Input: part model. Units: mm. Frame: model coordinates. Round coordinates to 2 decimals unless told otherwise and drop trailing zeros. Loops run counter-clockwise (first coordinate to the right, second up) from the corner with the lowest first, then second, coordinate; pieces in that order, holes last.
1) Section C-C, the plane y = 0.5. State how many separate pieces and enclosed holes the cut face has, and give its area (3 significant figures).
2) Ray query, line 1 along Z through (x, y) = (-41, 0.6); line 2 along X through (y, z) = (1.55, 247.5); line 3 along X through (y, z) = (1.05, 193.5). Return the intervals inside material, ascending.
3) First-contact query: pin 1 (0.5 mm diameter, centred on x = -77, y = 0.5, fed in from -Z); pin 2 (4 mm diameter, centred on x = -41.78, z = 255.06, fed in from -Y). Flat tips, straight axial feed; report the tip coordinate or a pass-through.
4) Section B-B, the plane z = 62. Return loops of the section in (x, y), and give its area (3 significant figures).
5) Section A-A, the plane x = -80. Return loops of the section in (y, z), and give its area (3 significant figures).
from build123d import *

# Parameters (mm, degrees)
SKETCH1_R        = 1.5
SKETCH1_R_2      = 1.600010398
SKETCH1_R_3      = 1.6
SKETCH1_R_4      = 1.35
EXTRUSION1_DEPTH = 1.6
FILLET1_R        = 1
FILLET2_R        = 4
FILLET3_R        = 3
FILLET4_R        = 3
FILLET5_R        = 2
FILLET6_R        = 2
FILLET7_R        = 3
FILLET8_R        = 3
FILLET9_R        = 2
FILLET10_R       = 2
FILLET11_R       = 3


with BuildPart() as part:
    # Sketch1 → Extrusion1 (new body)
    with BuildSketch(Plane(origin=(0, 0, 0), x_dir=(-1, 0, 0), z_dir=(0, 1, 0))):
        Polygon((59.775158519, 259.059874387), (56.775158519, 264.05987395), (36.775158519, 264.05987395), (36.775158519, 252.05987395), (18.755330752, 234.731117294), (21.527931817, 231.847944851), (10.275158581, 204.559863083), (7.271137723, 204.559863083), (7.157131709, 183.059873956), (7.157131709, 76.612413837), (10.15713177, 76.612413837), (21.409905007, 49.324332069), (18.637303942, 46.441159626), (36.657131709, 29.11240297), (36.657131709, 17.11240297), (56.657131709, 17.11240297), (59.657131709, 22.112402533), (78.657131709, 22.112402533), (97.657131709, 22.112402533), (100.657131709, 17.11240297), (120.657131709, 17.11240297), (120.657131709, 29.11240297), (138.676959475, 46.441159626), (135.90435841, 49.324332069), (147.157131647, 76.612413837), (150.157131709, 76.612413837), (150.157131709, 183.059873956), (150.275158519, 204.559863083), (147.275158457, 204.559863083), (136.022385221, 231.847944851), (138.794986286, 234.731117294), (120.775158519, 252.05987395), (120.775158519, 264.05987395), (100.775158519, 264.05987395), (97.775158519, 259.059874387), (78.657131709, 259.059874387), align=None)
        with Locations((55.657131647, 26.112401639)):
            Circle(SKETCH1_R, mode=Mode.SUBTRACT)
        with Locations((39.157131647, 33.112413837)):
            Circle(SKETCH1_R, mode=Mode.SUBTRACT)
        with Locations((53.657131709, 208.059873956)):
            Circle(SKETCH1_R_2, mode=Mode.SUBTRACT)
        with Locations((53.657131709, 158.059873956)):
            Circle(SKETCH1_R_2, mode=Mode.SUBTRACT)
        with Locations((17.157131647, 89.862401639)):
            Circle(SKETCH1_R_3, mode=Mode.SUBTRACT)
        with Locations((103.657131709, 158.059873956)):
            Circle(SKETCH1_R_2, mode=Mode.SUBTRACT)
        with Locations((41.775158457, 255.059863083)):
            Circle(SKETCH1_R, mode=Mode.SUBTRACT)
        with Locations((39.275158457, 248.059863083)):
            Circle(SKETCH1_R, mode=Mode.SUBTRACT)
        with Locations((10.775158457, 194.05987528)):
            Circle(SKETCH1_R_4, mode=Mode.SUBTRACT)
        with Locations((88.65713177, 26.862413837)):
            Circle(SKETCH1_R, mode=Mode.SUBTRACT)
        with Locations((115.65713177, 26.112413837)):
            Circle(SKETCH1_R, mode=Mode.SUBTRACT)
        with Locations((118.15713177, 33.112413837)):
            Circle(SKETCH1_R, mode=Mode.SUBTRACT)
        with Locations((140.15713177, 89.862401639)):
            Circle(SKETCH1_R_3, mode=Mode.SUBTRACT)
        with Locations((115.775158581, 255.059863083)):
            Circle(SKETCH1_R, mode=Mode.SUBTRACT)
        with Locations((88.775158581, 254.309863083)):
            Circle(SKETCH1_R, mode=Mode.SUBTRACT)
        with Locations((140.275158581, 191.30987528)):
            Circle(SKETCH1_R_3, mode=Mode.SUBTRACT)
        with Locations((146.775158581, 194.05987528)):
            Circle(SKETCH1_R_4, mode=Mode.SUBTRACT)
        with Locations((101.775158581, 255.05987528)):
            Circle(SKETCH1_R, mode=Mode.SUBTRACT)
        with Locations((118.275158581, 248.059863083)):
            Circle(SKETCH1_R, mode=Mode.SUBTRACT)
        with Locations((146.65713177, 87.112401639)):
            Circle(SKETCH1_R_4, mode=Mode.SUBTRACT)
        with Locations((101.65713177, 26.112401639)):
            Circle(SKETCH1_R, mode=Mode.SUBTRACT)
        with Locations((17.275158457, 191.30987528)):
            Circle(SKETCH1_R_3, mode=Mode.SUBTRACT)
        with Locations((55.775158457, 255.05987528)):
            Circle(SKETCH1_R, mode=Mode.SUBTRACT)
        with Locations((68.775158457, 254.309863083)):
            Circle(SKETCH1_R, mode=Mode.SUBTRACT)
        with Locations((10.657131647, 87.112401639)):
            Circle(SKETCH1_R_4, mode=Mode.SUBTRACT)
        with Locations((68.657131647, 26.862413837)):
            Circle(SKETCH1_R, mode=Mode.SUBTRACT)
        with Locations((41.657131647, 26.112413837)):
            Circle(SKETCH1_R, mode=Mode.SUBTRACT)
        with Locations((32.657131647, 39.362413837)):
            Circle(SKETCH1_R, mode=Mode.SUBTRACT)
        with Locations((124.775158581, 241.809863083)):
            Circle(SKETCH1_R, mode=Mode.SUBTRACT)
        with Locations((32.775158457, 241.809863083)):
            Circle(SKETCH1_R, mode=Mode.SUBTRACT)
        with Locations((103.657131709, 208.059873956)):
            Circle(SKETCH1_R_2, mode=Mode.SUBTRACT)
        with Locations((124.65713177, 39.362413837)):
            Circle(SKETCH1_R, mode=Mode.SUBTRACT)
    extrude(amount=EXTRUSION1_DEPTH)

    # Fillet1
    fillet1_edges = [part.edges().sort_by_distance(p)[0] for p in [
        (-97.775158519, 0.8, 259.059874387),
        (-97.657131709, 0.8, 22.112402533),
        (-59.657131709, 0.8, 22.112402533),
        (-59.775158519, 0.8, 259.059874387),
    ]]
    fillet(fillet1_edges, radius=FILLET1_R)

    # Fillet2
    fillet2_edges = [part.edges().sort_by_distance(p)[0] for p in [
        (-120.775158519, 0.8, 264.05987395),
        (-120.657131709, 0.8, 17.11240297),
        (-36.657131709, 0.8, 17.11240297),
        (-36.775158519, 0.8, 264.05987395),
    ]]
    fillet(fillet2_edges, radius=FILLET2_R)

    # Fillet3
    fillet3_edges = [part.edges().sort_by_distance(p)[0] for p in [
        (-120.775158519, 0.8, 252.05987395),
        (-120.657131709, 0.8, 29.11240297),
        (-36.657131709, 0.8, 29.11240297),
        (-36.775158519, 0.8, 252.05987395),
    ]]
    fillet(fillet3_edges, radius=FILLET3_R)

    # Fillet4
    fillet4_edges = [part.edges().sort_by_distance(p)[0] for p in [
        (-138.794986286, 0.8, 234.731117294),
    ]]
    fillet(fillet4_edges, radius=FILLET4_R)

    # Fillet5
    fillet5_edges = [part.edges().sort_by_distance(p)[0] for p in [
        (-136.022385221, 0.8, 231.847944851),
    ]]
    fillet(fillet5_edges, radius=FILLET5_R)

    # Fillet6
    fillet6_edges = [part.edges().sort_by_distance(p)[0] for p in [
        (-21.527931817, 0.8, 231.847944851),
    ]]
    fillet(fillet6_edges, radius=FILLET6_R)

    # Fillet7
    fillet7_edges = [part.edges().sort_by_distance(p)[0] for p in [
        (-18.755330752, 0.8, 234.731117294),
    ]]
    fillet(fillet7_edges, radius=FILLET7_R)

    # Fillet8
    fillet8_edges = [part.edges().sort_by_distance(p)[0] for p in [
        (-138.676959475, 0.8, 46.441159626),
        (-18.637303942, 0.8, 46.441159626),
    ]]
    fillet(fillet8_edges, radius=FILLET8_R)

    # Fillet9
    fillet9_edges = [part.edges().sort_by_distance(p)[0] for p in [
        (-21.409905007, 0.8, 49.324332069),
        (-135.90435841, 0.8, 49.324332069),
    ]]
    fillet(fillet9_edges, radius=FILLET9_R)

    # Fillet10
    fillet10_edges = [part.edges().sort_by_distance(p)[0] for p in [
        (-147.275158457, 0.8, 204.559863083),
        (-147.157131647, 0.8, 76.612413837),
        (-10.15713177, 0.8, 76.612413837),
        (-10.275158581, 0.8, 204.559863083),
    ]]
    fillet(fillet10_edges, radius=FILLET10_R)

    # Fillet11
    fillet11_edges = [part.edges().sort_by_distance(p)[0] for p in [
        (-150.275158519, 0.8, 204.559863083),
        (-7.157131709, 0.8, 76.612413837),
    ]]
    fillet(fillet11_edges, radius=FILLET11_R)


solid = part.part
Final values:
1. separate pieces: 1
1. enclosed holes: 32
1. area: 30,700 mm2
2. line 1: z = 17.11 to 24.76, 27.46 to 253.78, 256.34 to 264.06
2. line 2: x = -125.52 to -119.67, -116.88 to -40.67, -37.88 to -32.03
2. line 3: x = -150.21 to -148, -145.55 to -12, -9.55 to -7.21
3. pin 1: stops at z = 22.11
3. pin 2: stops at y = 0
4. outline: (-141.13, 0) - (-16.18, 0) - (-16.18, 1.6) - (-141.13, 1.6) - close
4. area: 200 mm2
5. outline: (0, 22.11) - (1.6, 22.11) - (1.6, 259.06) - (0, 259.06) - close
5. area: 379 mm2
